Geometry: final body of the model. Coordinates: model frame, mm. A direction names the side the tool comes from. Give positions to 0.01 mm unless a question says otherwise; leave off trailing zeros. Order: outer loops, then holes, each group sorted by start corner. A loop starts at its lowest first (then second) coordinate and runs counter-clockwise, first axis right, second up. Notation, with made-up numbers: (-28.5, 60) - (4.5, 60) arc R36 cw to (4.5, 96) - close; hole circle Ø8 at (17, 53). An arc over 180 degrees is marked (long way). Put each result on its own line as item: value. Start each with the question number.
1. First-contact query: P1, Ø4, axis at x = 9, y = 26.5, coming from the -Z side; P2, Ø1.4, axis at y = -2.5, z = -3, coming from the +X side (3 decimals); P3, Ø1.5, axis at x = 6.5, z = 1, coming from the +Y side; P4, Ø3, axis at x = 18.5, y = 11.5, coming from the -Z side. Flat tips, straight axial feed; report the tip coordinate or a pass-through.
2. Section A-A on x = 0. Count the separate pieces of the cut face and the enclosed holes in it, plus the area to 3 significant figures.
3. Ray query, line 1 along Y through (x, z) = (0, 2.4) (3 decimals); line 2 along Z through (x, y) = (46, 8.5) (3 decimals); line 3 along X through (y, z) = (17, 1.25). Return the intervals inside material, ascending. Write a range as from..to.
4. Mould query, pull axis X, two halves, no side actions, for faces 6 (the flat face through (-4, 41.4, 0)), 7 (the flat face through (25.4, 13, 2)), 8 (the flat face through (-41.275, -3, -2)). Classes: pulls with the +X half, pulls with the -X half, needs draft (parallel to the pull), parting line crosses it, or undercut.
5. Section D-D on y = 38.5. Return the cut outline in (x, z) (1 decimal), plus the area to 3 significant figures.
6. Section C-C on y = 15. Return the cut outline in (x, z) (1 decimal), plus the area to 3 significant figures.
7. Set-up query: faces 1 (the flat face through (-1, -6.35, 1)), 2 (the cylindrical face through (0.908, 41.265, -2.348)), 3 (the cylindrical face through (0.698, 31.742, -2.348)), 4 (the flat face through (0, 17.78, 2)), 5 (the flat face through (41.275, -3, -2)). Return all of +Z, -Z, +X, -X, +Y, -Y with unobstructed straight access to the full face (end or side cutting, diameter ignored); none if empty.
8. Section B-B on z = -3. Return the cut outline in (x, y) (3 decimals).
Autodesk Inventor part; units mm, degrees
ref_plane "YZ Plane" through (0, 0, 0) normal (1, 0, 0) x (0, 1, 0)
ref_plane "XZ Plane" through (0, 0, 0) normal (0, 1, 0) x (-1, 0, 0)
ref_plane "XY Plane" through (0, 0, 0) normal (0, 0, 1) x (1, 0, 0)
sketch "Sketch2" plane through (0, 0, 0) normal (0, 0, 1) x (1, 0, 0)
  arc A0 (31.75, 0) -> (-31.75, 0) centre (0, 0) ccw
  arc A1 (41.275, 0) -> (-41.275, 0) centre (0, 0) ccw
  line L0 (-41.275, 0) -> (-31.75, 0)
  line L1 (31.75, 0) -> (41.275, 0)
  arc A2 (50.8, 0) -> (-50.8, 0) centre (0, 0) ccw
  line L2 (-50.8, 0) -> (-41.275, 0)
  line L3 (41.275, 0) -> (50.8, 0)
  line L4 (-31.75, 0) -> (31.75, 0)
  line L5 (0, 0) -> (0, 31.75) construction
  line L6 (0, 8.255) -> (25.4, 8.255)
  line L7 (25.4, 8.255) -> (25.4, 17.78)
  line L8 (25.4, 17.78) -> (0, 17.78)
  line L9 (0, 17.78) -> (-25.4, 17.78)
  line L10 (-25.4, 17.78) -> (-25.4, 8.255)
  line L11 (-25.4, 8.255) -> (0, 8.255)
  dimension "d2" = 63.5
  dimension "d3" = 9.525
  dimension "d4" = 9.525
  dimension "d5" = 25.4
  dimension "d6" = 8.255
  dimension "d7" = 9.525
extrude "Extrusion3" add sketch "Sketch2" along normal blind 3.175
extrude "Extrusion4" add sketch "Sketch2" against normal blind 4.7625 contours A0 L0 A1 L1
sketch "Sketch5" plane through (0, 0, 3.175) normal (0, 0, 1) x (1, 0, 0)
  arc A0 (31.75, 0) -> (-31.75, 0) centre (0, 0) ccw
  line L0 (-25.4, 17.78) -> (25.4, 17.78)
  line L1 (0, 31.75) -> (0, 17.78) construction
  point P0 (0, 24.765)
hole "Hole2" at (0, 24.765, 3.175) direction (0, 0, -1) diameter 5.1054 end through all
sketch "Sketch8" plane through (-50.8, 0, 3.175) normal (0, -1, 0) x (1, 0, 0)
  line L0 (101.6, -3.175) -> (101.6, 0)
  line L1 (101.6, 0) -> (101.6, -3.175)
  line L2 (92.075, -3.175) -> (101.6, -3.175)
  line L3 (101.6, -3.175) -> (92.075, -3.175)
  line L4 (92.075, -7.9375) -> (82.55, -7.9375)
  line L5 (92.075, -3.175) -> (92.075, -7.9375)
  line L6 (92.075, -7.9375) -> (82.55, -7.9375)
  line L7 (82.55, -3.175) -> (82.55, -7.9375)
  line L8 (82.55, -7.9375) -> (82.55, -3.175)
  line L9 (82.55, -3.175) -> (19.05, -3.175)
  line L10 (19.05, -3.175) -> (19.05, -7.9375)
  line L11 (19.05, -3.175) -> (19.05, -7.9375)
  line L12 (9.525, -7.9375) -> (92.075, -7.9375)
  line L13 (19.05, -7.9375) -> (9.525, -7.9375)
  line L14 (9.525, -3.175) -> (9.525, -7.9375)
  line L15 (9.525, -7.9375) -> (9.525, -3.175)
  line L16 (0, -3.175) -> (9.525, -3.175)
  line L17 (9.525, -3.175) -> (0, -3.175)
  line L18 (0, -3.175) -> (0, 0)
  line L19 (0, -3.175) -> (0, 0)
  line L20 (0, 0) -> (101.6, 0)
  point P0 (50.8, -3.175)
extrude "Extrusion6" add sketch "Sketch8" along normal blind 6.35 contours L2 L5 L4 L7 L9 L10 L12 L14 L16 L18 L20 L0
equation "\"d2\" = insideDiameterOfRing"
equation "\"d3\" = innerRingWidth"
equation "\"d4\" = outerRingWidth"
equation "\"d5\" = halfWidthForPryBar"
equation "\"d7\" = depthForPryBar"
equation "\"d12\" = bottomFlat"
equation "\"d14\" = bottomSupport"
equation "\"insideDiameterOfRing\" = 63.5"
equation "\"wallThicknessOfRing\" = 9.525"
equation "\"outsideDiameterOfRing\" = insideDiameterOfRing + 2 * wallThicknessOfRing"
equation "\"widthForPryBar\" = 50.8"
equation "\"outerRingWidth\" = 9.525"
equation "\"innerRingWidth\" = 9.525"
equation "\"halfWidthForPryBar\" = 0.5 * widthForPryBar"
equation "\"distanceFromEdgeToPryBar\" = 8.255"
equation "\"totalHeightOfPart\" = 19.05"
equation "\"topPartHeight\" = 6.35"
equation "\"lowerPartHeight\" = totalHeightOfPart - topPartHeight"
equation "\"depthForPryBar\" = 9.525"
equation "\"bottomFlat\" = 3.175"
equation "\"bottomSupport\" = 4.7625"
properties part number "dRingHolderBottom" material "PBT Plastic"
Resolved:
1. P1: z = 0
1. P2: x = 41.275
1. P3: y = 50.47
1. P4: through
2. separate pieces: 3
2. enclosed holes: 0
2. area: 180 mm^2
3. line 1: -6.35..8.255, 17.78..22.212, 27.318..50.8
3. line 2: 0..3.175
3. line 3: -47.87..-25.4, 25.4..47.87
4. face 6: needs draft
4. face 7: undercut
4. face 8: pulls with the -X half
5. outline: (-33.1, 0) - (-14.9, 0) - (-14.9, -4.8) - (14.9, -4.8) - (14.9, 0) - (33.1, 0) - (33.1, 3.2) - (-33.1, 3.2) - close
5. area: 352 mm^2
6. outline: (-48.5, 0) - (-38.5, 0) - (-38.5, -4.8) - (-28, -4.8) - (-28, 0) - (-25.4, 0) - (-25.4, 3.2) - (-48.5, 3.2) - close; (25.4, 0) - (28, 0) - (28, -4.8) - (38.5, -4.8) - (38.5, 0) - (48.5, 0) - (48.5, 3.2) - (25.4, 3.2) - close
6. area: 247 mm^2
7. face 1: +Z, -Z, +X, -X, -Y
7. face 2: -Z, +Y
7. face 3: -Z, -Y
7. face 4: +Z, -Z
7. face 5: -Z, +X, +Y, -Y
8. outline: (-41.275, -6.35) - (-31.75, -6.35) - (-31.75, 0) arc R31.75 cw to (31.75, 0) - (31.75, -6.35) - (41.275, -6.35) - (41.275, 0) arc R41.275 ccw to (-41.275, 0) - close
